from build123d import *

# Parameters (mm, degrees)
PAD_DEPTH            = 62
POCKET_DEPTH         = 213.922356
SKETCH002_R          = 20
POCKET001_DEPTH      = 213.922356
SKETCH003_R          = 10
POCKET002_DEPTH      = 102.531483
POCKET002_DEPTH_BACK = 0.001
PAD001_DEPTH         = 60
SKETCH005_R          = 20
POCKET003_DEPTH      = 60
POCKET004_DEPTH      = 212.557512
SKETCH007_W          = 150
SKETCH007_H          = 20
POCKET005_DEPTH      = 74.846137
FILLET_R             = 20


with BuildPart() as part:
    # Sketch → Pad (new body, symmetric)
    with BuildSketch(Plane.XZ):
        Polygon((0, 0), (200, 0), (200, -25), (10.355339, -25), (-67.175144, -102.530483), (-84.852814, -84.852814), align=None)
    extrude(amount=PAD_DEPTH, both=True)

    # Sketch001 (on DatumPlane) → Pocket (cut, through all)
    with BuildSketch(Plane(origin=(0, 0, 0), x_dir=(0.707107, 0, 0.707107), z_dir=(-0.707107, 0, 0.707107))):
        with BuildLine():
            Line((-130, 62), (0, 62))
            Line((0, 62), (-90.013078, 38.726454))
            ThreePointArc((-90.013078, 38.726454), (-120, 0), (-90.013078, -38.726454))
            Line((0, -62), (-90.013078, -38.726454))
            Line((0, -62), (-130, -62))
            Line((-130, -62), (-130, 62))
        make_face()
    extrude(amount=-POCKET_DEPTH, mode=Mode.SUBTRACT)

    # Sketch002 (on DatumPlane) → Pocket001 (cut, through all)
    with BuildSketch(Plane(origin=(0, 0, 0), x_dir=(0.707107, 0, 0.707107), z_dir=(-0.707107, 0, 0.707107))):
        with Locations((-80, 0)):
            Circle(SKETCH002_R)
    extrude(amount=-POCKET001_DEPTH, mode=Mode.SUBTRACT)

    # Sketch003 → Pocket002 (cut, two sides)
    with BuildSketch(Plane.XY) as pocket002_sk:
        with Locations((25, 40)):
            Circle(SKETCH003_R)
        with Locations((175, 40)):
            Circle(SKETCH003_R)
        with Locations((175, -40)):
            Circle(SKETCH003_R)
        with Locations((25, -40)):
            Circle(SKETCH003_R)
    extrude(amount=-POCKET002_DEPTH, mode=Mode.SUBTRACT)
    extrude(pocket002_sk.sketch, amount=POCKET002_DEPTH_BACK, mode=Mode.SUBTRACT)

    # Sketch004 (on DatumPlane) → Pad001 (join)
    with BuildSketch(Plane(origin=(0, -56, 0), x_dir=(0.965926, 0.258819, 0), z_dir=(0.224144, -0.836516, 0.5))):
        with BuildLine():
            Line((140, 79.999939), (140, 0))
            Line((140, 0), (60, 0))
            Line((60, 0), (60, 80.000001))
            ThreePointArc((79.999999, 100), (65.857864, 94.142136), (60, 80.000001))
            Line((79.999999, 100), (120, 100))
            ThreePointArc((140, 79.999939), (134.142157, 94.142114), (120, 100))
        make_face()
    extrude(amount=-PAD001_DEPTH)

    # Sketch005 (on DatumPlane) → Pocket003 (cut)
    with BuildSketch(Plane(origin=(0, -56, 0), x_dir=(0.965926, 0.258819, 0), z_dir=(0.224144, -0.836516, 0.5))):
        with Locations((100, 70)):
            Circle(SKETCH005_R)
    extrude(amount=-POCKET003_DEPTH, mode=Mode.SUBTRACT)

    # Sketch006 (on DatumPlane) → Pocket004 (cut, through all)
    with BuildSketch(Plane(origin=(0, 0, 0), x_dir=(-0.258819, 0.965926, 0), z_dir=(0.965926, 0.258819, 0))):
        Polygon((-40.23544, 0), (6.300459, 80.60254), (37.477373, 62.60254), (1.33378, 0), align=None)
    extrude(amount=POCKET004_DEPTH, mode=Mode.SUBTRACT)

    # Sketch007 → Pocket005 (cut, through all)
    with BuildSketch(Plane.XZ):
        with Locations((90, -35)):
            Rectangle(SKETCH007_W, SKETCH007_H)
    extrude(amount=-POCKET005_DEPTH, mode=Mode.SUBTRACT)

    # Fillet
    fillet_edges = [part.edges().sort_by_distance(p)[0] for p in [
        (200, -62, -12.5),
        (200, 62, -12.5),
    ]]
    fillet(fillet_edges, radius=FILLET_R)


solid = part.part
Input: part model. Units: mm. Frame: model coordinates. A direction names the side the tool comes from. Coordinates: 2 decimals unless noted, no trailing zeros. Loops run counter-clockwise (first coordinate to the right, second up) from the corner with the lowest first, then second, coordinate; pieces in that order, holes last. Notation, with made-up numbers: (3, 44) -> (11, 44) arc R13 ccw to (11, 53) -> close; hole circle Ø8 at (80.25, 55). An arc over 180 degrees is marked (long way). Write item = value, one per line. Start each with the question number.
Item 1: Cut plane C-C, the plane x = 3. Return loops of the section in (y, z), plus the area to 3 significant figures.
Item 2: First-contact query: P1, Ø5, axis at x = -37, z = -71.5, coming from the -Y side; P2, Ø16, axis at x = 175, y = -40, coming from the -Z side; P3, Ø2, axis at y = -8, z = -38, coming from the -X side; P4, Ø6, axis at x = 99, z = 21.5, coming from the -Y side. Flat tips, straight axial feed; report the tip coordinate or a pass-through.
Item 3: Cut plane D-D, the plane x = 77.5. Count the separate pieces of the cut face and the enclosed holes in it, plus the area to 3 significant figures.
Item 4: Mould query, pull axis X, two halves, no side actions, for faces 4 (the face through (99, -1, 0)), 5 (the face through (73.788, 38.239, 16.755)), 6 (the face through (-21.832, -50.526, -40.926)). Classes: pulls with the +X half, pulls with the -X half, needs draft (parallel to the pull), parting line crosses it, or undercut.
Item 5: Reachability of faces 1 (the face through (107, -1, -25)), 2 (the face through (128.655, 4.772, 32.168)), 3 (the face through (29.614, -48.872, -12.325)) from +Z, -Z, +X, -X, +Y, -Y: full face, straight path, thin tool, end or side. Return the list, or none.
Item 6: Cut plane B-B, the plane z = -22. Return loops of the section in (x, y), plus the area to 3 significant figures.
Item 7: Material intervals for line 1 (Y direction, x = 25, z = -15.25); line 2 (X direction, y = 40, z = -19.25); line 3 (Y direction, x = 179, z = -14), sorted ascending.
Item 8: Cut plane A-A, the plane x = 175. Return loops of the section in (y, z).
Ans:
q1.outline = (-62, -3) -> (-56.63, -32.36) -> (56.63, -32.36) -> (62, -3) -> (62, 0) -> (-62, 0) -> close
q1.area = 3,850 mm²
q2.P1 = -42.81
q2.P2 = through
q2.P3 = -39
q2.P4 = -18.59
q3.separate_pieces = 3
q3.enclosed_holes = 0
q3.area = 4,220 mm²
q4.face_4 = needs draft
q4.face_5 = undercut
q4.face_6 = pulls with the -X half
q5.face_1 = -Z, +X, +Y, -Y
q5.face_2 = +Z, +X, +Y
q5.face_3 = +Z, -Z
q6.outline = (-22, -53.96) -> (22, -62) -> (180, -62) arc R20 ccw to (200, -42) -> (200, 42) arc R20 ccw to (180, 62) -> (22, 62) -> (-22, 53.96) -> close; hole circle Ø20 at (25, -40); hole circle Ø20 at (25, 40); hole circle Ø20 at (175, -40); hole circle Ø20 at (175, 40)
q6.area = 25,700 mm²
q7.line_1 = -62 to -50, -30 to 30, 50 to 62
q7.line_2 = -19.25 to 15, 35 to 165, 185 to 200
q7.line_3 = -62 to -49.17, -30.83 to 30.83, 49.17 to 62
q8.outline = (-62, -25) -> (-50, -25) -> (-50, 0) -> (-62, 0) -> close; (-30, -25) -> (30, -25) -> (30, 0) -> (-30, 0) -> close; (50, -25) -> (62, -25) -> (62, 0) -> (50, 0) -> close
